Geometry check sheet. Reference: the model listing, model coordinates, mm. Give positions to 0.01 mm unless a question says otherwise; leave off trailing zeros. Write each loop counter-clockwise with the first axis right and the second up, starting at its lowest first coordinate (ties: lowest second). Pieces come first, ordered by that corner, then holes. Notation, with made-up numbers: (64.5, -29.75) -> (86.5, -29.75) arc R14 cw to (86.5, -20.75) -> close; hole circle Ø5 at (-12, -24). An arc over 180 degrees is marked (long way). Write item = value, one per line. Start each with the question number.
1. Cross-section at B-B, the plane y = -65. Record the cut outline in (x, z).
2. Depth check by flat-ended pin: P1, Ø12, axis at x = -14.5, y = 32.5, coming from the -Z side; P2, Ø2.5, axis at x = 54, y = -54, coming from the +Z side; P3, Ø0.6, axis at x = 50.5, z = 1.5, coming from the +Y side. Enter the tip coordinate at first touch or a pass-through.
3. Cross-section at C-C, the plane x = -47. Record the cut outline in (y, z).
4. Thickness scan on line 1 along Y through (x, z) = (0, 1.3); line 2 along Y through (x, z) = (22, 1); line 3 along X through (y, z) = (11, 1.4). Record the ranges inside material, lowest first.
5. Cross-section at D-D, the plane y = -18. Record the cut outline in (x, z), plus the area to 3 significant figures.
6. Cross-section at A-A, the plane x = -62. Record the cut outline in (y, z), plus the area to 3 significant figures.
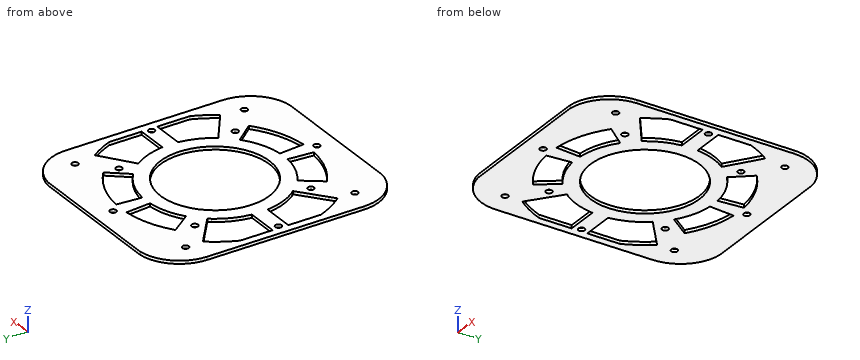
```python
from build123d import *

# Parameters (mm, degrees)
SKETCH1_W           = 90
SKETCH1_H           = 100
SKETCH1_H_2         = 22
SKETCH1_W_2         = 24
BOSS_EXTRUDE1_DEPTH = 2
CUT_EXTRUDE1_DEPTH  = 10
CUT_EXTRUDE2_DEPTH  = 10
SKETCH4_R           = 30
CUT_EXTRUDE3_DEPTH  = 10
CUT_EXTRUDE4_DEPTH  = 10
CUT_EXTRUDE5_DEPTH  = 10
BOSS_EXTRUDE3_START = -2
SKETCH8_R           = 30
SKETCH8_R_2         = 28
BOSS_EXTRUDE3_DEPTH = 2
BOSS_EXTRUDE5_DEPTH = 2
BOSS_EXTRUDE6_DEPTH = 2
SKETCH11_R          = 34.778777804
CUT_EXTRUDE6_DEPTH  = 10
SKETCH12_R          = 2
CUT_EXTRUDE7_DEPTH  = 10


with BuildPart() as part:
    # Sketch1 → Boss-Extrude1 (new body)
    with BuildSketch(Plane.XY):
        Rectangle(SKETCH1_W, SKETCH1_H)
        with Locations((0, 61)):
            Rectangle(SKETCH1_W, SKETCH1_H_2)
        with Locations((57, 0)):
            Rectangle(SKETCH1_W_2, SKETCH1_H)
        with BuildLine():
            Line((45, 50), (69, 50))
            ThreePointArc((69, 50), (61.278820596, 65.667804287), (45, 72))
            Line((45, 72), (45, 50))
        make_face()
        with BuildLine():
            ThreePointArc((45, -72), (61.83891888, -66.278820596), (69, -50))
            Line((69, -50), (45, -50))
            Line((45, -50), (45, -72))
        make_face()
        with Locations((0, -61)):
            Rectangle(SKETCH1_W, SKETCH1_H_2)
        with BuildLine():
            Line((-45, -72), (-45, -50))
            Line((-45, -50), (-69, -50))
            ThreePointArc((-69, -50), (-61.278820596, -65.667804287), (-45, -72))
        make_face()
        with Locations((-57, 0)):
            Rectangle(SKETCH1_W_2, SKETCH1_H)
        with BuildLine():
            Line((-69, 50), (-45, 50))
            Line((-45, 50), (-45, 72))
            ThreePointArc((-45, 72), (-61.83891888, 66.278820596), (-69, 50))
        make_face()
    extrude(amount=BOSS_EXTRUDE1_DEPTH)

    # Sketch2 → Cut-Extrude1 (cut)
    with BuildSketch(Plane.XY.offset(2)):
        with BuildLine():
            Line((-60.760739313, 25.787593916), (-64, 15.649215929))
            Line((-64, 15.649215929), (-64, 5))
            Line((-64, 5), (-43.724760028, 5))
            ThreePointArc((-43.724760028, 5), (-41.091915324, 15.757827722), (-35.856683042, 25.517698186))
            Line((-35.856683042, 25.517698186), (-56.217391304, 40.007560722))
            ThreePointArc((-56.217391304, 40.007560722), (-60.52773874, 33.126920216), (-64, 25.787593916))
            Line((-64, 25.787593916), (-60.760739313, 25.787593916))
        make_face()
        with BuildLine():
            Line((-64, -5), (-64, -25.787593916))
            ThreePointArc((-64, -25.787593916), (-60.52773874, -33.126920216), (-56.217391304, -40.007560722))
            Line((-56.217391304, -40.007560722), (-35.856683042, -25.517698186))
            ThreePointArc((-35.856683042, -25.517698186), (-41.091915324, -15.757827722), (-43.724760028, -5))
            Line((-43.724760028, -5), (-64, -5))
        make_face()
        with BuildLine():
            Line((-35.483097289, 48.383362913), (-26.026680798, 35.488963441))
            ThreePointArc((-26.026680798, 35.488963441), (-15.448259809, 41.209293956), (-3.716315379, 43.852521472))
            Line((-3.716315379, 43.852521472), (-5.066584601, 59.785698294))
            ThreePointArc((-5.066584601, 59.785698294), (-21.061160661, 56.182092446), (-35.483097289, 48.383362913))
        make_face()
        with BuildLine():
            ThreePointArc((64, 25.787593916), (60.52773874, 33.126920216), (56.217391304, 40.007560722))
            Line((56.217391304, 40.007560722), (35.856683042, 25.517698186))
            ThreePointArc((35.856683042, 25.517698186), (41.091915324, 15.757827722), (43.724760028, 5))
            Line((43.724760028, 5), (64, 5))
            Line((64, 5), (64, 25.787593916))
        make_face()
        with BuildLine():
            Line((-26.026680798, -35.488963441), (-35.483097289, -48.383362913))
            ThreePointArc((-35.483097289, -48.383362913), (-21.061160661, -56.182092446), (-5.066584601, -59.785698294))
            Line((-5.066584601, -59.785698294), (-3.716315379, -43.852521472))
            ThreePointArc((-3.716315379, -43.852521472), (-15.448259809, -41.209293956), (-26.026680798, -35.488963441))
        make_face()
        with BuildLine():
            ThreePointArc((56.217391304, -40.007560722), (60.52773874, -33.126920216), (64, -25.787593916))
            Line((64, -25.787593916), (64, -5))
            Line((64, -5), (43.724760028, -5))
            ThreePointArc((43.724760028, -5), (41.091915324, -15.757827722), (35.856683042, -25.517698186))
            Line((35.856683042, -25.517698186), (56.217391304, -40.007560722))
        make_face()
        with BuildLine():
            Line((27.916279909, 34.022580083), (38.059254795, 46.384190458))
            ThreePointArc((38.059254795, 46.384190458), (22.588514074, 55.585600941), (5.084745763, 59.784156434))
            Line((5.084745763, 59.784156434), (3.729636503, 43.851390526))
            ThreePointArc((3.729636503, 43.851390526), (16.568566174, 40.771770312), (27.916279909, 34.022580083))
        make_face()
        with BuildLine():
            Line((3.729636503, -43.851390526), (5.084745763, -59.784156434))
            ThreePointArc((5.084745763, -59.784156434), (22.588514074, -55.585600941), (38.059254795, -46.384190458))
            Line((38.059254795, -46.384190458), (27.916279909, -34.022580083))
            ThreePointArc((27.916279909, -34.022580083), (16.568566174, -40.771770312), (3.729636503, -43.851390526))
        make_face()
    extrude(amount=-CUT_EXTRUDE1_DEPTH, mode=Mode.SUBTRACT)

    # Sketch3 → Cut-Extrude2 (cut)
    with BuildSketch(Plane.XY.offset(2)):
        Polygon((-64, 25.787593916), (-64, 15.649215929), (-60.760739313, 25.787593916), align=None)
    extrude(amount=-CUT_EXTRUDE2_DEPTH, mode=Mode.SUBTRACT)

    # Sketch4 → Cut-Extrude3 (cut)
    with BuildSketch(Plane(origin=(0, 0, 0), x_dir=(-1, 0, 0), z_dir=(0, 0, -1))):
        Circle(SKETCH4_R)
    extrude(amount=-CUT_EXTRUDE3_DEPTH, mode=Mode.SUBTRACT)

    # Sketch6 → Cut-Extrude4 (cut)
    with BuildSketch(Plane.XY.offset(2)):
        Polygon((-35.856683042, -25.517698186), (-56.217391304, -40.007560722), (-50.280397209, -40.007560722), (-34.257403731, -27.258240508), align=None)
        Polygon((-50.280397209, 40.007560722), (-56.217391304, 40.007560722), (-35.856683042, 25.517698186), (-34.257403731, 27.258240508), align=None)
        Polygon((-50.280397209, -40.007560722), (-56.217391304, -40.007560722), (-53.993303971, -42.96187992), align=None)
        Polygon((-53.993303971, 42.96187992), (-56.217391304, 40.007560722), (-50.280397209, 40.007560722), align=None)
    extrude(amount=-CUT_EXTRUDE4_DEPTH, mode=Mode.SUBTRACT)

    # Sketch7 → Cut-Extrude5 (cut)
    with BuildSketch(Plane.XY.offset(2)):
        Polygon((-32.560271117, 27.267561972), (-24.823321267, 33.603144582), (-18.487738656, 25.866194731), (-26.224688507, 19.530612121), align=None)
        Polygon((27.827762823, 32.155388995), (19.915267174, 26.040455421), (26.030200748, 18.127959772), (33.942696396, 24.242893346), align=None)
        Polygon((33.988304577, -25.549058378), (27.336365779, -18.082351592), (19.869658993, -24.734290389), (26.521597791, -32.200997176), align=None)
        Polygon((-26.126682472, -33.612215797), (-18.478667441, -27.169555937), (-24.921327301, -19.521540905), (-32.569342333, -25.964200766), align=None)
    extrude(amount=-CUT_EXTRUDE5_DEPTH, mode=Mode.SUBTRACT)

    # Sketch8 → Boss-Extrude3 (add)
    with BuildSketch(Plane.XY.offset(2).offset(BOSS_EXTRUDE3_START)):
        Circle(SKETCH8_R)
        Circle(SKETCH8_R_2, mode=Mode.SUBTRACT)
    extrude(amount=BOSS_EXTRUDE3_DEPTH)

    # Sketch9 → Boss-Extrude5 (add)
    with BuildSketch(Plane(origin=(0, 0, 0), x_dir=(-1, 0, 0), z_dir=(0, 0, -1))):
        Polygon((32.694861491, 27.157349491), (26.359278881, 19.420399641), (18.487738656, 25.866194731), (24.823321267, 33.603144582), align=None)
        Polygon((32.547632539, -25.945912516), (26.104972678, -33.593927547), (18.478667441, -27.169555937), (24.921327301, -19.521540905), align=None)
        Polygon((-27.336365779, -18.082351592), (-34.046734551, -25.614645193), (-26.580027765, -32.266583991), (-19.869658993, -24.734290389), align=None)
        Polygon((-27.829205352, 32.153522415), (-19.916709703, 26.038588842), (-26.030200748, 18.127959772), (-33.942696396, 24.242893346), align=None)
        with BuildLine():
            Line((-45, 72), (0, 72))
            Line((0, 72), (0, 77))
            Line((0, 77), (-45, 77))
            ThreePointArc((-45, 77), (-62.132690852, 68.062391868), (-69, 50))
            ThreePointArc((-69, 50), (-61.278820596, 65.667804287), (-45, 72))
        make_face()
        with BuildLine():
            Line((0, 77), (0, 72))
            Line((0, 72), (45, 72))
            ThreePointArc((45, 72), (61.278820596, 65.667804287), (69, 50))
            ThreePointArc((69, 50), (62.132690852, 68.062391868), (45, 77))
            Line((45, 77), (0, 77))
        make_face()
        with BuildLine():
            ThreePointArc((45, -77), (62.132690852, -68.062391868), (69, -50))
            ThreePointArc((69, -50), (61.278820596, -65.667804287), (45, -72))
            Line((45, -72), (0, -72))
            Line((0, -72), (0, -77))
            Line((0, -77), (45, -77))
        make_face()
        with BuildLine():
            ThreePointArc((-45, -72), (-61.278820596, -65.667804287), (-69, -50))
            ThreePointArc((-69, -50), (-62.132690852, -68.062391868), (-45, -77))
            Line((-45, -77), (0, -77))
            Line((0, -77), (0, -72))
            Line((0, -72), (-45, -72))
        make_face()
    extrude(amount=-BOSS_EXTRUDE5_DEPTH)

    # Sketch10 → Boss-Extrude6 (add)
    with BuildSketch(Plane(origin=(0, 0, 0), x_dir=(-1, 0, 0), z_dir=(0, 0, -1))):
        Polygon((-27.829205352, 32.153522415), (-27.827762823, 32.155388995), (-19.915267174, 26.040455421), (-19.916709703, 26.038588842), align=None)
        Polygon((26.104972678, -33.593927547), (26.126682472, -33.612215797), (32.568924212, -25.964697113), (32.547214419, -25.946408862), align=None)
    extrude(amount=-BOSS_EXTRUDE6_DEPTH)

    # Sketch11 → Cut-Extrude6 (cut)
    with BuildSketch(Plane(origin=(0, 0, 0), x_dir=(-1, 0, 0), z_dir=(0, 0, -1))):
        Circle(SKETCH11_R)
    extrude(amount=-CUT_EXTRUDE6_DEPTH, mode=Mode.SUBTRACT)

    # Sketch12 → Cut-Extrude7 (cut)
    with BuildSketch(Plane.XY.offset(2)):
        with Locations((0, -65)):
            Circle(SKETCH12_R)
        with Locations((62, 0)):
            Circle(SKETCH12_R)
        with Locations((-62, 0)):
            Circle(SKETCH12_R)
        with Locations((0, 65)):
            Circle(SKETCH12_R)
        with Locations((-37.029437252, 37.029437252)):
            Circle(SKETCH12_R)
        with Locations((-54, 54)):
            Circle(SKETCH12_R)
        with Locations((54, 54)):
            Circle(SKETCH12_R)
        with Locations((37.029437252, 37.029437252)):
            Circle(SKETCH12_R)
        with Locations((-54, -54)):
            Circle(SKETCH12_R)
        with Locations((-37.029437252, -37.029437252)):
            Circle(SKETCH12_R)
        with Locations((37.029437252, -37.029437252)):
            Circle(SKETCH12_R)
        with Locations((54, -54)):
            Circle(SKETCH12_R)
    extrude(amount=-CUT_EXTRUDE7_DEPTH, mode=Mode.SUBTRACT)


solid = part.part
```
Answers:
q1.outline = (-64.49, 0) -> (-2, 0) -> (-2, 2) -> (-64.49, 2) -> close; (2, 0) -> (64.49, 0) -> (64.49, 2) -> (2, 2) -> close
q2.P1 = 0
q2.P2 = through
q2.P3 = 75.86
q3.outline = (-76.69, 0) -> (-37.4, 0) -> (-37.4, 2) -> (-76.69, 2) -> close; (-5, 0) -> (5, 0) -> (5, 2) -> (-5, 2) -> close; (37.4, 0) -> (76.69, 0) -> (76.69, 2) -> (37.4, 2) -> close
q4.line_1 = -77 to -67, -63 to -34.78, 34.78 to 63, 67 to 77
q4.line_2 = -77 to -55.82, -38.12 to -26.94, 26.94 to 38.12, 55.82 to 77
q4.line_3 = -69 to -64, -42.61 to -32.99, 32.99 to 42.61, 64 to 69
q5.outline = (-69, 0) -> (-64, 0) -> (-64, 2) -> (-69, 2) -> close; (-40.16, 0) -> (-29.76, 0) -> (-29.76, 2) -> (-40.16, 2) -> close; (29.76, 0) -> (40.16, 0) -> (40.16, 2) -> (29.76, 2) -> close; (64, 0) -> (69, 0) -> (69, 2) -> (64, 2) -> close
q5.area = 61.6 mm^2
q6.outline = (-68.21, 0) -> (-30.28, 0) -> (-30.28, 2) -> (-68.21, 2) -> close; (-5, 0) -> (-2, 0) -> (-2, 2) -> (-5, 2) -> close; (2, 0) -> (5, 0) -> (5, 2) -> (2, 2) -> close; (30.28, 0) -> (68.21, 0) -> (68.21, 2) -> (30.28, 2) -> close
q6.area = 164 mm^2
